Design review of the part built by this model. Coordinates are the model's own, in mm. A direction names the side the tool comes from. Round coordinates to 2 decimals unless told otherwise and drop trailing zeros. Order: outer loops, then holes, each group sorted by start corner. A loop starts at its lowest first (then second) coordinate and runs counter-clockwise, first axis right, second up. Notation, with made-up numbers: (69, 42.5) - (112, 42.5) arc R18 cw to (112, 46.5) - close; hole circle Ø6 at (-23, -11). An arc over 180 degrees is marked (long way). Write item = value, one per line.
from build123d import *

# Parameters (mm, degrees)
SKETCH1_R               = 72.5
BOSS_EXTRUDE1_DEPTH     = 10
BOSS_EXTRUDE2_DEPTH     = 15
SKETCH3_R               = 3
CUT_EXTRUDE1_DEPTH      = 10
MIRROR3_COPY_1_SKETCH_R = 3
MIRROR3_COPY_1_DEPTH    = 10


with BuildPart() as part:
    # Sketch1 → Boss-Extrude1 (new body)
    with BuildSketch(Plane(origin=(0, 0, 0), x_dir=(1, 0, 0), z_dir=(0, 1, 0))):
        with Locations(Location((0, 0, 0), (0, 0, 270))):
            Circle(SKETCH1_R)
    extrude(amount=BOSS_EXTRUDE1_DEPTH)

    # Sketch2 → Boss-Extrude2 (add)
    with BuildSketch(Plane.XZ):
        with BuildLine():
            Line((-22.246900451, 62.865113828), (22.246900451, 62.865113828))
            ThreePointArc((22.246900451, 62.865113828), (29.317968263, 59.93618164), (32.246900451, 52.865113828))
            Line((32.246900451, 52.865113828), (32.246900451, 15.536222894))
            Line((32.246900451, 15.536222894), (-32.246900451, 15.536222894))
            Line((-32.246900451, 15.536222894), (-32.246900451, 52.865113828))
            ThreePointArc((-32.246900451, 52.865113828), (-29.317968263, 59.93618164), (-22.246900451, 62.865113828))
        make_face()
    boss_extrude2 = extrude(amount=BOSS_EXTRUDE2_DEPTH)

    # Mirror1: Boss-Extrude2 across plane
    add(boss_extrude2.mirror(Plane.XY))

    # Sketch3 → Cut-Extrude1 (cut)
    with BuildSketch(Plane.XZ):
        with Locations(Location((-49.458347743, 36.215950375, 0), (0, 0, 270))):
            Circle(SKETCH3_R)
        with Locations(Location((-49.458347743, 17.215950375, 0), (0, 0, 270))):
            Circle(SKETCH3_R)
    cut_extrude1 = extrude(amount=-CUT_EXTRUDE1_DEPTH, mode=Mode.SUBTRACT)

    # Mirror2: Cut-Extrude1 across plane
    add(cut_extrude1.mirror(Plane.XY), mode=Mode.SUBTRACT)

    # Mirror3: Cut-Extrude1 across plane
    add(cut_extrude1.mirror(Plane(origin=(0, 0, 0), x_dir=(0, 0, 1), z_dir=(1, 0, 0))), mode=Mode.SUBTRACT)

    # Mirror3 copy 1 sketch → Mirror3 copy 1 (cut)
    with BuildSketch(Plane(origin=(0, 0, 0), x_dir=(-1, 0, 0), z_dir=(0, -1, 0))):
        with Locations(Location((-49.458347743, 36.215950375, 0), (0, 0, 270))):
            Circle(MIRROR3_COPY_1_SKETCH_R)
        with Locations(Location((-49.458347743, 17.215950375, 0), (0, 0, 270))):
            Circle(MIRROR3_COPY_1_SKETCH_R)
    extrude(amount=-MIRROR3_COPY_1_DEPTH, mode=Mode.SUBTRACT)


solid = part.part
1) We need section C-C on z = 61. Write out the cut boundary in (x, y), and give its area (3 significant figures).
Findings:
outline = (-39.18, 0) - (-28.06, 0) - (-28.06, -15) - (28.06, -15) - (28.06, 0) - (39.18, 0) - (39.18, 10) - (-39.18, 10) - close
area = 1,630 mm^2
2) Clearance check with flat-ended pins moving along their axes: pin 1 Ø8 at (x, y) = (19, 2) entering from +Z; pin 2 Ø7.5 at (x, y) = (1.5, -9) entering from -Z; pin 3 Ø8 at (y, z) = (-4.5, 28.5) entering from -X. State where each tip first meets the part, or that it passes through.
Findings:
pin_1 = 70.93
pin_2 = -62.87
pin_3 = -32.25
3) For faces 1 (the flat face through (0, -7, -62.865)), 2 (the flat face through (32.247, -7, -34)), 3 (the flat face through (0, -7, 15.536)), 4 (the cylindrical face through (-29.395, -7.395, 59.858)), 5 (the flat face through (-32.247, -7, 34)), list the 3-axis set-ups (+Z, -Z, +X, -X, +Y, -Y) from which the entire face can be reached by the end or side of a thin tool; tool diameter is ignored.
Findings:
face_1 = -Z, +X, -X, -Y
face_2 = +Z, -Z, +X, -Y
face_3 = +X, -X, -Y
face_4 = +Z, -X, -Y
face_5 = +Z, -Z, -X, -Y
4) To check wall thickness, follow L1, parallel to Z at x = -13, y = -2; L2, parallel to Y at x = 38, z = -7.5; L3, parallel to X at y = -0.75, z = 18.5. State the ranges of each line that lie inside material, in increasing order. Write a range as from..to.
Findings:
L1 = -62.87..-15.54, 15.54..62.87
L2 = 0..10
L3 = -32.25..32.25
5) We need section D-D on x = 16. Write out the cut boundary in (y, z), and give its area (3 significant figures).
Findings:
outline = (-15, -62.87) - (0, -62.87) - (0, -70.71) - (10, -70.71) - (10, 70.71) - (0, 70.71) - (0, 62.87) - (-15, 62.87) - (-15, 15.54) - (0, 15.54) - (0, -15.54) - (-15, -15.54) - close
area = 2,830 mm^2
6) The part is to be moulded in two halves that separate along Z. For faces 6 (the cylindrical face through (-52.12, 4.93, 15.83)), 7 (the flat face through (0, -15, -40)), 8 (the cylindrical face through (29.24, -7.395, -60.014)), say which applies: released by +Z, released by -Z, zero draft, split by the parting line, or undercut.
Findings:
face_6 = undercut
face_7 = zero draft
face_8 = released by -Z
7) We need section B-B on x = 0. Write out the cut boundary in (y, z).
Findings:
outline = (-15, -62.87) - (0, -62.87) - (0, -72.5) - (10, -72.5) - (10, 72.5) - (0, 72.5) - (0, 62.87) - (-15, 62.87) - (-15, 15.54) - (0, 15.54) - (0, -15.54) - (-15, -15.54) - close
8) We need section A-A on y = -3.75. Write out the cut boundary in (x, z), and give its area (3 significant figures).
Findings:
outline = (-32.25, -52.87) arc R10 ccw to (-22.25, -62.87) - (22.25, -62.87) arc R10 ccw to (32.25, -52.87) - (32.25, -15.54) - (-32.25, -15.54) - close; (-32.25, 15.54) - (32.25, 15.54) - (32.25, 52.87) arc R10 ccw to (22.25, 62.87) - (-22.25, 62.87) arc R10 ccw to (-32.25, 52.87) - close
area = 6,020 mm^2
